```python
from build123d import *

# Parameters (mm, degrees)
F0_W     = 7
F0_H     = 65.71
F1_DEPTH = 10
F2_W     = 3.25
F2_H     = 3.71
F3_DEPTH = 10
F5_DEPTH = 10
F6_W     = 6
F6_H     = 12.01
F7_DEPTH = 7
F9_DEPTH = 10


with BuildPart() as f1:
    # F0 (on Front) → F1 (new body)
    with BuildSketch(Plane.XZ):
        Rectangle(F0_W, F0_H)
    extrude(amount=-F1_DEPTH)

    # F2 (on face) → F3 (cut, through all)
    with BuildSketch(Plane.XZ):
        with Locations((-1.875, 31)):
            Rectangle(F2_W, F2_H)
        with Locations((1.875, 31)):
            Rectangle(F2_W, F2_H)
    extrude(amount=-F3_DEPTH, mode=Mode.SUBTRACT)

    # F4 (on face) → F5 (cut, through all)
    with BuildSketch(Plane.XZ):
        with BuildLine():
            Line((-1.75, -12.155), (-1.75, -18.155))
            ThreePointArc((-1.75, -18.155), (0, -19.905), (1.75, -18.155))
            Line((1.75, -18.155), (1.75, -12.155))
            ThreePointArc((1.75, -12.155), (0, -10.405), (-1.75, -12.155))
        make_face()
        with BuildLine():
            Line((-1.75, 2.845), (-1.75, -3.155))
            ThreePointArc((-1.75, -3.155), (0, -4.905), (1.75, -3.155))
            Line((1.75, -3.155), (1.75, 2.845))
            ThreePointArc((1.75, 2.845), (0, 4.595), (-1.75, 2.845))
        make_face()
    extrude(amount=-F5_DEPTH, mode=Mode.SUBTRACT)

    # F6 (on face) → F7 (cut, through all)
    with BuildSketch(Plane.YZ.offset(3.5)):
        with Locations((3, 26.85)):
            Rectangle(F6_W, F6_H)
    extrude(amount=-F7_DEPTH, mode=Mode.SUBTRACT)

    # F8 (on face) → F9 (cut)
    with BuildSketch(Plane(origin=(0, 0, -32.855), x_dir=(1, 0, 0), z_dir=(0, 0, -1))):
        with BuildLine():
            ThreePointArc((0, -3.5), (-1.06066, -6.06066), (1.5, -5))
            ThreePointArc((1.5, -5), (1.06066, -3.93934), (0, -3.5))
        make_face()
    extrude(amount=-F9_DEPTH, mode=Mode.SUBTRACT)


solid = f1.part
```
Source: CAD feature listing. Evaluate the final solid. Frame: model axes, mm. A direction names the side the tool comes from. Coordinates: 2 decimals unless noted, no trailing zeros. Order: outer loops, then holes, each group sorted by start corner. A loop starts at its lowest first (then second) coordinate and runs counter-clockwise, first axis right, second up. Notation, with made-up numbers: M -39,-23 L -16,-23 A16 cw -16,6 Z; hole C -3.5,45 d11. An arc over 180 degrees is marked long. Write each question's results on one line, items separated by ' | '. Start each with the question number.
1) Access query for faces 1 (the face through (0, 6, 25)), 2 (the face through (-2, 8, 29.145)), 3 (the face through (-0.038, 4.93, -19.905)), 4 (the face through (2, 8, 29.145)). Directions: +Z, -Z, +X, -X, +Y, -Y. A direction counts if a zero-diameter tool reaches every point of the face in a straight line with its end or side. Return the directions, or none.
2) Section query A-A (y = 1). Return the cut outline in (x, z) (3 decimals), plus the area to 3 significant figures.
3) Section query B-B (z = -11.5). Return the cut outline in (x, y), plus the area to 3 significant figures.
4) Draft query along X for faces 5 (the face through (0.038, 4.93, 4.595)), 6 (the face through (-3.5, 5, -2)), 7 (the face through (2, 10, 0)). Return one class per face: released by +X, released by -X, zero draft, split by the parting line, or undercut.
5) Contact query for flat-ended pins moving along their axis: pin 1 Ø4 at (x, y) = (0, 5) entering from -Z (3 decimals); pin 2 Ø1.8 at (x, y) = (0, 1.5) entering from +Z (3 decimals); pin 3 Ø2.5 at (x, y) = (0, 5) entering from -Z (3 decimals); pin 4 Ø1 at (x, y) = (-1.5, 8) entering from +Z (3 decimals). Output: stop coordinate, or through.
6) Section query C-C (z = 24). Return the cut outline in (x, y).
7) Line query: line 1 (X direction, y = 5, z = -29.75); line 2 (Z direction, x = 1.5, y = 8.25) (3 decimals); line 3 (Z direction, x = 2.5, y = 2) (3 decimals). Output: solid intervals per line, ascending. Write a range as from..to.
Answers:
1) face 1: +Z, +X, -X, -Y | face 2: +Z, -X, +Y, -Y | face 3: +Y, -Y | face 4: +Z, +X, +Y, -Y
2) outline: M -3.5,-32.855 L 3.5,-32.855 L 3.5,20.845 L -3.5,20.845 Z; hole M -1.75,-18.155 A1.75 ccw 1.75,-18.155 L 1.75,-12.155 A1.75 ccw -1.75,-12.155 Z; hole M -1.75,-3.155 A1.75 ccw 1.75,-3.155 L 1.75,2.845 A1.75 ccw -1.75,2.845 Z | area: 315 mm^2
3) outline: M -3.5,0 L -1.62,0 L -1.62,10 L -3.5,10 Z; M 1.62,0 L 3.5,0 L 3.5,10 L 1.62,10 Z | area: 37.5 mm^2
4) face 5: undercut | face 6: released by -X | face 7: zero draft
5) pin 1: stops at z = -32.855 | pin 2: stops at z = 20.845 | pin 3: stops at z = -22.855 | pin 4: stops at z = 29.145
6) outline: M -3.5,6 L 3.5,6 L 3.5,10 L -3.5,10 Z
7) line 1: x = -3.5..-1.5, 1.5..3.5 | line 2: z = -32.855..-19.056, -11.254..-4.056, 3.746..29.145 | line 3: z = -32.855..20.845
